```python
from build123d import *

# Parameters (mm, degrees)
SKETCH1_W           = 4
SKETCH1_H           = 8
SKETCH1_H_2         = 4
SKETCH1_W_2         = 8
BOSS_EXTRUDE1_DEPTH = 70
FILLET1_R           = 1
SKETCH3_R           = 1.75
CUT_EXTRUDE2_DEPTH  = 70
CUT_EXTRUDE3_REACH  = 72.83
SKETCH2_R           = 1.75


with BuildPart() as part:
    # Sketch1 → Boss-Extrude1 (new body)
    with BuildSketch(Plane.XY):
        with Locations((-5.272021997, 1.455882353)):
            Rectangle(SKETCH1_W, SKETCH1_H)
        with Locations((-5.272021997, -4.544117647)):
            Rectangle(SKETCH1_W, SKETCH1_H_2)
        with Locations((0.727978003, -4.544117647)):
            Rectangle(SKETCH1_W_2, SKETCH1_H_2)
    extrude(amount=BOSS_EXTRUDE1_DEPTH)

    # Fillet1
    fillet1_edges = [part.edges().sort_by_distance(p)[0] for p in [
        (-3.272021997, -2.544117647, 35),
    ]]
    fillet(fillet1_edges, radius=FILLET1_R)

    # Sketch3 → Cut-Extrude2 (cut)
    with BuildSketch(Plane(origin=(-3.272021997, 0, 0), x_dir=(0, 0, -1), z_dir=(1, 0, 0))):
        with Locations(Location((-55, 1.955882353, 0), (0, 0, 90))):
            Circle(SKETCH3_R)
        with Locations(Location((-15, 1.955882353, 0), (0, 0, 90))):
            Circle(SKETCH3_R)
        with Locations(Location((-35, 1.955882353, 0), (0, 0, 90))):
            Circle(SKETCH3_R)
    extrude(amount=-CUT_EXTRUDE2_DEPTH, mode=Mode.SUBTRACT)

    # Sketch2 → Cut-Extrude3 (cut, up to next)
    with BuildSketch(Plane(origin=(0, -2.544117647, 0), x_dir=(1, 0, 0), z_dir=(0, 1, 0)), mode=Mode.PRIVATE) as cut_extrude3_sk1:
        with Locations(Location((1.227978003, -50, 0), (0, 0, 270))):
            Circle(SKETCH2_R)
    cut_extrude3_tool1 = extrude(cut_extrude3_sk1.sketch, amount=-CUT_EXTRUDE3_REACH, mode=Mode.PRIVATE) & part.part
    # Sketch2 → Cut-Extrude3 (cut, up to next)
    with BuildSketch(Plane(origin=(0, -2.544117647, 0), x_dir=(1, 0, 0), z_dir=(0, 1, 0)), mode=Mode.PRIVATE) as cut_extrude3_sk2:
        with Locations(Location((1.227978003, -20, 0), (0, 0, 270))):
            Circle(SKETCH2_R)
    cut_extrude3_tool2 = extrude(cut_extrude3_sk2.sketch, amount=-CUT_EXTRUDE3_REACH, mode=Mode.PRIVATE) & part.part
    add(cut_extrude3_tool1.solids().sort_by_distance((1.227978, -2.544118, 50))[0], mode=Mode.SUBTRACT)
    add(cut_extrude3_tool2.solids().sort_by_distance((1.227978, -2.544118, 20))[0], mode=Mode.SUBTRACT)


solid = part.part
```
For this review, take the finished solid that the model builds, in its own axes (mm). A direction names the side the tool comes from. Give positions to 0.01 mm unless a question says otherwise; leave off trailing zeros. Write each loop counter-clockwise with the first axis right and the second up, starting at its lowest first coordinate (ties: lowest second). Pieces come first, ordered by that corner, then holes.
Item 1: Insertion check: P1, Ø5.5, axis at y = 0.5, z = 51, coming from the +X side; P2, Ø5.5, axis at x = 0, z = 42.5, coming from the +Y side; P3, Ø3, axis at x = 1.23, z = 20, coming from the +Y side; P4, Ø3, axis at y = -0.5, z = 54.5, coming from the +X side. Each pin has a flat end and moves straight along its axis. Give the tip position at first contact, or say it passes through.
Item 2: Take a section at C-C (z = 50.5). Give the boundary of the cut face in (x, y), and give its area (3 significant figures).
Item 3: Take a section at B-B (z = 5). Give the boundary of the cut face in (x, y).
Item 4: Take a section at A-A (z = 15). Give the boundary of the cut face in (x, y), and give its area (3 significant figures).
Item 5: The part is to be moulded in two halves that separate along X. For faces 1 (the face through (4.728, -5, 35)), 2 (the face through (1.3, -4.52, 18.25)), 3 (the face through (-5, 5.456, 35)), 4 (the face through (0.558, -4.516, 51.617)), say which applies: +X half, -X half, draft (parallel to the pull), parting line (faces both ways), or undercut.
Item 6: Machinability: for faces 5 (the face through (-5.24, 1.58, 33.29)), 6 (the face through (-3.272, 0, 35)), which of the approach directions +Z, -Z, +X, -X, +Y, -Y give a long, thin tool a straight path to every point of the face, cutting with its end or side? Answer none if there is none.
Item 7: Wall thickness on probe 1 along X at (y, z) = (-3.35, 50); probe 2 along X at (y, z) = (2, 9.5); probe 3 along Y at (x, z) = (-2.25, 58.5): over which ranges is each line inside the solid? List them lowest first.
Established:
1. P1: stops at x = -2.98
1. P2: stops at y = -2.42
1. P3: passes through
1. P4: stops at x = -3.16
2. outline: (-7.27, -6.54) - (-0.45, -6.54) - (-0.45, -2.54) - (-2.27, -2.54) arc R1 cw to (-3.27, -1.54) - (-3.27, 5.46) - (-7.27, 5.46) - close; (2.91, -6.54) - (4.73, -6.54) - (4.73, -2.54) - (2.91, -2.54) - close
2. area: 66.8 mm2
3. outline: (-7.27, -6.54) - (4.73, -6.54) - (4.73, -2.54) - (-2.27, -2.54) arc R1 cw to (-3.27, -1.54) - (-3.27, 5.46) - (-7.27, 5.46) - close
4. outline: (-7.27, -6.54) - (4.73, -6.54) - (4.73, -2.54) - (-2.27, -2.54) arc R1 cw to (-3.27, -1.54) - (-3.27, 0.21) - (-7.27, 0.21) - close; (-7.27, 3.71) - (-3.27, 3.71) - (-3.27, 5.46) - (-7.27, 5.46) - close
4. area: 66.2 mm2
5. face 1: +X half
5. face 2: undercut
5. face 3: draft
5. face 4: undercut
6. face 5: +X, -X
6. face 6: +Z, -Z, +X, +Y
7. probe 1: x = -7.27 to -0.52, 2.98 to 4.73
7. probe 2: x = -7.27 to -3.27
7. probe 3: y = -6.54 to -2.54
